Check sheet for the modelled part. Datum: model origin and axes. Units: mm. A direction names the side the tool comes from. Give positions to 0.01 mm unless a question says otherwise; leave off trailing zeros. Loops run counter-clockwise (first coordinate to the right, second up) from the corner with the lowest first, then second, coordinate; pieces in that order, holes last. Notation, with made-up numbers: (-7, 72.25) - (52, 72.25) arc R14 cw to (52, 84.25) - close; hole circle Ø6 at (85.25, 35). An arc over 180 degrees is marked (long way). Use CSV: the item, a comma, the result in double quotes.
from build123d import *

# Parameters (mm, degrees)
PAD008_DEPTH    = 11
POCKET005_DEPTH = 9
SKETCH019_W     = 6.25
SKETCH019_H     = 58.5
PAD009_DEPTH    = 4
SKETCH020_W     = 6.25
SKETCH020_H     = 44.9
POCKET008_DEPTH = 2
SKETCH021_W     = 5
SKETCH021_H     = 86.8
SKETCH021_H_2   = 52
PAD010_DEPTH    = 10
SKETCH024_W     = 62
SKETCH024_H     = 2
POCKET011_DEPTH = 162.801
POCKET012_DEPTH = 4
SKETCH027_W     = 2.8
SKETCH027_H     = 2.4
SKETCH032_W     = 2.8
SKETCH032_H     = 1.6
SKETCH030_W     = 2.8
SKETCH030_H     = 2.4
SKETCH033_W     = 2.8
SKETCH033_H     = 1.6
SKETCH029_W     = 2.8
SKETCH029_H     = 2.4
SKETCH034_W     = 2.8
SKETCH034_H     = 1.6
SKETCH028_W     = 2.8
SKETCH028_H     = 2.4
SKETCH044_W     = 2.8
SKETCH044_H     = 1.6
CHAMFER_SIZE    = 1
SKETCH053_R     = 1.2
POCKET013_DEPTH = 4
SKETCH057_R     = 1.2
POCKET015_DEPTH = 3
SKETCH072_R     = 1.8
SKETCH072_W     = 10
SKETCH072_H     = 2
POCKET024_DEPTH = 3
SKETCH073_W     = 2
SKETCH073_H     = 38.5
POCKET025_DEPTH = 1.2
CHAMFER005_SIZE = 1.4


with BuildPart() as part:
    # Sketch015 → Pad008 (new body)
    with BuildSketch(Plane.XY):
        with BuildLine():
            Line((-54.5, 81.4), (80, 81.4))
            ThreePointArc((88, 73.4), (85.656854, 79.056854), (80, 81.4))
            Line((88, 73.4), (88, 19))
            ThreePointArc((80, 11), (85.656854, 13.343146), (88, 19))
            Line((76, 11), (80, 11))
            ThreePointArc((76, 11), (65.039845, 6.460155), (60.5, -4.5))
            Line((60.5, -75.4), (60.5, -4.5))
            ThreePointArc((54.5, -81.4), (58.742641, -79.642641), (60.5, -75.4))
            Line((54.5, -81.4), (-54.5, -81.4))
            ThreePointArc((-60.5, -75.4), (-58.742641, -79.642641), (-54.5, -81.4))
            Line((-60.5, -75.4), (-60.5, 75.4))
            ThreePointArc((-54.5, 81.4), (-58.742641, 79.642641), (-60.5, 75.4))
        make_face()
    extrude(amount=PAD008_DEPTH)

    # Sketch016 (on Face14 of Pad008) → Pocket005 (cut)
    with BuildSketch(Plane.XY.offset(11)):
        with BuildLine():
            Line((-54.7, 78.6), (80.2, 78.6))
            ThreePointArc((85.2, 73.6), (83.735534, 77.135534), (80.2, 78.6))
            Line((85.2, 73.6), (85.2, 18.8))
            ThreePointArc((80.2, 13.8), (83.735534, 15.264466), (85.2, 18.8))
            Line((76.2, 13.8), (80.2, 13.8))
            ThreePointArc((76.2, 13.8), (63.118525, 8.381475), (57.7, -4.7))
            Line((57.7, -75.6), (57.7, -4.7))
            ThreePointArc((54.7, -78.6), (56.82132, -77.72132), (57.7, -75.6))
            Line((54.7, -78.6), (-54.7, -78.6))
            ThreePointArc((-57.7, -75.6), (-56.82132, -77.72132), (-54.7, -78.6))
            Line((-57.7, -75.6), (-57.7, 75.6))
            ThreePointArc((-54.7, 78.6), (-56.82132, 77.72132), (-57.7, 75.6))
        make_face()
    extrude(amount=-POCKET005_DEPTH, mode=Mode.SUBTRACT)

    # Sketch019 (on Face27 of Pocket005) → Pad009 (join)
    with BuildSketch(Plane.XY.offset(2)):
        with Locations((-13.875, 43.25)):
            Rectangle(SKETCH019_W, SKETCH019_H)
        with Locations((81.875, 43.25)):
            Rectangle(SKETCH019_W, SKETCH019_H)
    extrude(amount=PAD009_DEPTH)

    # Sketch020 (on Face37 of Pad009) → Pocket008 (cut)
    with BuildSketch(Plane.XY.offset(6)):
        with Locations((-13.875, 43.25)):
            Rectangle(SKETCH020_W, SKETCH020_H)
        with Locations((81.875, 43.25)):
            Rectangle(SKETCH020_W, SKETCH020_H)
    extrude(amount=-POCKET008_DEPTH, mode=Mode.SUBTRACT)

    # Sketch021 (on Face27 of Pocket008) → Pad010 (join)
    with BuildSketch(Plane.XY.offset(2)):
        with Locations((-47, 5)):
            Rectangle(SKETCH021_W, SKETCH021_H)
        with Locations((47, -12.4)):
            Rectangle(SKETCH021_W, SKETCH021_H_2)
    extrude(amount=PAD010_DEPTH)

    # Sketch024 (on Face6 of Pad010) → Pocket011 (cut, through all)
    with BuildSketch(Plane.XZ.offset(81.4)):
        with Locations((0, 10)):
            Rectangle(SKETCH024_W, SKETCH024_H)
    extrude(amount=-POCKET011_DEPTH, mode=Mode.SUBTRACT)

    # Sketch025 (on Face5 of Pocket011) → Pocket012 (cut)
    with BuildSketch(Plane.XY.offset(11)):
        with BuildLine():
            Line((-54.5, 81.4), (-44.5, 81.4))
            Line((-44.5, 81.4), (-44.5, 78.6))
            Line((-54.7, 78.6), (-44.5, 78.6))
            ThreePointArc((-54.7, 78.6), (-56.82132, 77.72132), (-57.7, 75.6))
            Line((-57.7, 65.4), (-57.7, 75.6))
            Line((-57.7, 65.4), (-60.5, 65.4))
            Line((-60.5, 65.4), (-60.5, 75.4))
            ThreePointArc((-54.5, 81.4), (-58.742641, 79.642641), (-60.5, 75.4))
        make_face()
        with BuildLine():
            Line((70, 81.4), (80, 81.4))
            ThreePointArc((88, 73.4), (85.656854, 79.056854), (80, 81.4))
            Line((88, 73.4), (88, 63.4))
            Line((88, 63.4), (85.2, 63.4))
            Line((85.2, 73.4), (85.2, 63.4))
            ThreePointArc((85.2, 73.4), (83.676955, 77.076955), (80, 78.6))
            Line((70, 78.6), (80, 78.6))
            Line((70, 78.6), (70, 81.4))
        make_face()
        with BuildLine():
            Line((-60.5, -65.4), (-57.7, -65.4))
            Line((-57.7, -75.6), (-57.7, -65.4))
            ThreePointArc((-57.7, -75.6), (-56.82132, -77.72132), (-54.7, -78.6))
            Line((-44.5, -78.6), (-54.7, -78.6))
            Line((-44.5, -78.6), (-44.5, -81.4))
            Line((-44.5, -81.4), (-54.5, -81.4))
            ThreePointArc((-60.5, -75.4), (-58.742641, -79.642641), (-54.5, -81.4))
            Line((-60.5, -75.4), (-60.5, -65.4))
        make_face()
        with BuildLine():
            Line((57.7, -65.4), (60.5, -65.4))
            Line((60.5, -65.4), (60.5, -75.4))
            ThreePointArc((54.5, -81.4), (58.742641, -79.642641), (60.5, -75.4))
            Line((54.5, -81.4), (44.5, -81.4))
            Line((44.5, -81.4), (44.5, -78.6))
            Line((54.7, -78.6), (44.5, -78.6))
            ThreePointArc((54.7, -78.6), (56.82132, -77.72132), (57.7, -75.6))
            Line((57.7, -65.4), (57.7, -75.6))
        make_face()
    extrude(amount=-POCKET012_DEPTH, mode=Mode.SUBTRACT)

    # Sketch027 (on Face35 of Pocket012) → SubtractiveLoft section 0
    with BuildSketch(Plane.XZ.offset(65.4)):
        with Locations((-59.1, 8.2)):
            Rectangle(SKETCH027_W, SKETCH027_H)
    # Sketch032 (on DatumPlane) → SubtractiveLoft section 1
    with BuildSketch(Plane.XZ.offset(64.8)):
        with Locations((-59.1, 8.2)):
            Rectangle(SKETCH032_W, SKETCH032_H)
    loft(mode=Mode.SUBTRACT)

    # Sketch030 (on Face35 of Pocket012) → SubtractiveLoft001 section 0
    with BuildSketch(Plane.XZ.offset(65.4)):
        with Locations((59.1, 8.2)):
            Rectangle(SKETCH030_W, SKETCH030_H)
    # Sketch033 (on DatumPlane) → SubtractiveLoft001 section 1
    with BuildSketch(Plane.XZ.offset(64.8)):
        with Locations((59.1, 8.2)):
            Rectangle(SKETCH033_W, SKETCH033_H)
    loft(mode=Mode.SUBTRACT)

    # Sketch029 → SubtractiveLoft002 section 0
    with BuildSketch(Plane(origin=(0, 65.4, 0), x_dir=(-1, 0, 0), z_dir=(0, 1, 0))):
        with Locations((59.1, 8.2)):
            Rectangle(SKETCH029_W, SKETCH029_H)
    # Sketch034 (on DatumPlane) → SubtractiveLoft002 section 1
    with BuildSketch(Plane(origin=(0, 64.8, 0), x_dir=(-1, 0, 0), z_dir=(0, 1, 0))):
        with Locations((59.1, 8.2)):
            Rectangle(SKETCH034_W, SKETCH034_H)
    loft(mode=Mode.SUBTRACT)

    # Sketch028 → SubtractiveLoft003 section 0
    with BuildSketch(Plane(origin=(0, 63.4, 0), x_dir=(-1, 0, 0), z_dir=(0, 1, 0))):
        with Locations((-86.6, 8.2)):
            Rectangle(SKETCH028_W, SKETCH028_H)
    # Sketch044 (on DatumPlane) → SubtractiveLoft003 section 1
    with BuildSketch(Plane(origin=(0, 62.8, 0), x_dir=(-1, 0, 0), z_dir=(0, 1, 0))):
        with Locations((-86.6, 8.2)):
            Rectangle(SKETCH044_W, SKETCH044_H)
    loft(mode=Mode.SUBTRACT)

    # Chamfer
    chamfer_edges = [part.edges().sort_by_distance(p)[0] for p in [
        (-10.75, 20.8, 5),
        (-10.75, 65.7, 5),
        (78.75, 65.7, 5),
        (78.75, 20.8, 5),
    ]]
    chamfer(chamfer_edges, length=CHAMFER_SIZE)

    # Sketch053 (on Face74 of Chamfer) → Pocket013 (cut)
    with BuildSketch(Plane.XY.offset(6)):
        with Locations((-14, 69.1)):
            Circle(SKETCH053_R)
        with Locations((-14, 17.4)):
            Circle(SKETCH053_R)
        with Locations((82, 17.4)):
            Circle(SKETCH053_R)
        with Locations((82, 69.1)):
            Circle(SKETCH053_R)
    extrude(amount=-POCKET013_DEPTH, mode=Mode.SUBTRACT)

    # Sketch057 (on Face87 of Pocket013) → Pocket015 (cut)
    with BuildSketch(Plane.XZ.offset(81.4)):
        with Locations((-2, 4)):
            Circle(SKETCH057_R)
        with Locations((2, 4)):
            Circle(SKETCH057_R)
    extrude(amount=-POCKET015_DEPTH, mode=Mode.SUBTRACT)

    # Sketch072 (on Face19 of Pocket015) → Pocket024 (cut)
    with BuildSketch(Plane.XZ.offset(-78.6)):
        with Locations((63, 6)):
            Circle(SKETCH072_R)
        with Locations((75, 6)):
            Rectangle(SKETCH072_W, SKETCH072_H)
    extrude(amount=-POCKET024_DEPTH, mode=Mode.SUBTRACT)

    # Sketch073 (on Face85 of Pocket024) → Pocket025 (cut)
    with BuildSketch(Plane.XY.offset(4)):
        with Locations((-11.75, 43.25)):
            Rectangle(SKETCH073_W, SKETCH073_H)
    extrude(amount=-POCKET025_DEPTH, mode=Mode.SUBTRACT)

    # Chamfer005
    chamfer005_edges = [part.edges().sort_by_distance(p)[0] for p in [
        (0, -81.4, 9),
        (0, 81.4, 9),
    ]]
    chamfer(chamfer005_edges, length=CHAMFER005_SIZE)


solid = part.part
1. Sectioned sample at C-C, the plane x = 18. Record the boundary of the cut face in (y, z), and give its area (3 significant figures).
Completed:
outline,"(-81.4, 0) - (81.4, 0) - (81.4, 7.6) - (80, 9) - (78.6, 9) - (78.6, 2) - (-78.6, 2) - (-78.6, 9) - (-80, 9) - (-81.4, 7.6) - close"
area,"363 mm²"
2. Scan lines: line 1 along Y through (x, z) = (-14, 3.5); line 2 along X through (y, z) = (69.1, 3.15); line 3 along Y through (x, z) = (2, 7). Record each from-to range of solid material in increasing order.
Completed:
line 1,"y = -81.4 to -78.6, 14 to 16.2, 18.6 to 67.9, 70.3 to 72.5, 78.6 to 81.4"
line 2,"x = -60.5 to -57.7, -17 to -15.2, -12.8 to -10.75, 78.75 to 80.8, 83.2 to 85, 85.2 to 88"
line 3,"y = -81.4 to -78.6, 78.6 to 81.4"
3. Set-up check for faces 1 (the face through (47, 13.6, 7)), 2 (the face through (-58.789, -79.596, 3.451)): record each of +Z, -Z, +X, -X, +Y, -Y from which the full face is reachable in a straight line by a thin tool's end or side.
Completed:
face 1,"+Z"
face 2,"+Z, -Z, -X, -Y"
4. Go/stop test with flat-tipped pins: pin 1 Ø1.2 at (x, y) = (82.5, 69) entering from +Z; pin 2 Ø7 at (x, y) = (-13.5, 37) entering from +Z; pin 3 Ø1 at (x, z) = (82, 5.5) entering from +Y. Record where each tip stops, or that it passes through.
Completed:
pin 1,"stops at z = 2"
pin 2,"stops at z = 4"
pin 3,"stops at y = 81.26"
5. Sectioned sample at D-D, the plane y = -27. Record the boundary of the cut face in (x, z).
Completed:
outline,"(-60.5, 0) - (60.5, 0) - (60.5, 11) - (57.7, 11) - (57.7, 2) - (49.5, 2) - (49.5, 12) - (44.5, 12) - (44.5, 2) - (-44.5, 2) - (-44.5, 12) - (-49.5, 12) - (-49.5, 2) - (-57.7, 2) - (-57.7, 11) - (-60.5, 11) - close"
6. Release check for a two-part mould opening along Y. For faces 3 (the face through (-12.5, 17.4, 6)), 4 (the face through (65.16, 6.58, 5.42)), 5 (the face through (85.719, 78.994, 3.451)) record: released by +Y, released by -Y, zero draft, split by the parting line, or undercut.
Completed:
face 3,"undercut"
face 4,"released by -Y"
face 5,"released by +Y"
7. Sectioned sample at B-B, the plane x = 63. Record the boundary of the cut face in (y, z).
Completed:
outline,"(3.94, 0) - (81.4, 0) - (81.4, 4.2) - (78.6, 4.2) - (78.6, 2) - (8.26, 2) - (8.26, 11) - (3.94, 11) - close; (78.6, 7.8) - (81.4, 7.8) - (81.4, 11) - (78.6, 11) - close"
8. Sectioned sample at A-A, the plane y = 44.5. Record the boundary of the cut face in (x, z), and give its area (3 significant figures).
Completed:
outline,"(-60.5, 0) - (88, 0) - (88, 11) - (85.2, 11) - (85.2, 2) - (85, 2) - (85, 4) - (78.75, 4) - (78.75, 2) - (-10.75, 2) - (-10.75, 2.8) - (-12.75, 2.8) - (-12.75, 4) - (-17, 4) - (-17, 2) - (-44.5, 2) - (-44.5, 12) - (-49.5, 12) - (-49.5, 2) - (-57.7, 2) - (-57.7, 11) - (-60.5, 11) - close"
area,"420 mm²"
